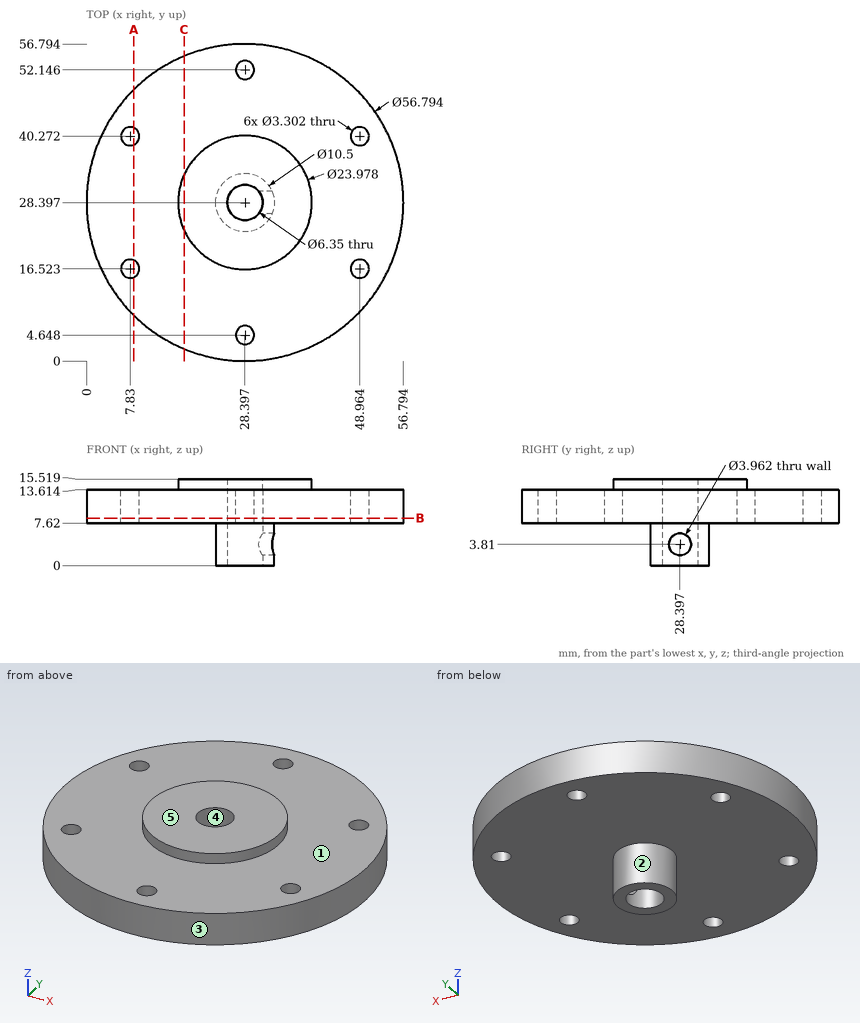
Part print with two shaded views. Sizes in mm from the minimum x, y, z corner. A direction names the side the tool comes from. Give positions to 0.01 mm unless a question says otherwise; leave off trailing zeros. Write each loop counter-clockwise with the first axis right and the second up, starting at its lowest first coordinate (ties: lowest second). Pieces come first, ordered by that corner, then holes.
1) Probe L1, parallel to Z at x = 20, y = 26; L2, parallel to Z at x = 35.5, y = 5 (1 decimal); L3, parallel to X at y = 27.5, z = 6.75 (1 decimal). List the from-to ranges inside material, lowest first.
Resolved:
L1: z = 7.62 to 15.52
L2: z = 7.6 to 13.6
L3: x = 23.2 to 25.4, 31.4 to 33.6
2) Two-plate mould, pull along Y, no slides. Class the marked faces 3, 4 and 5: released by +Y, released by -Y, zero draft, split by the parting line, or undercut.
Resolved:
face 3: split by the parting line
face 4: undercut
face 5: zero draft
3) Which spindle directions (+Z, -Z, +X, -X, +Y, -Y) get a long thin tool onto all of the face, cutting with end or side? Do the marked faces 1 and 2. Say none if no direction does.
Resolved:
face 1: +Z
face 2: -Z
4) Pin check, flat tips, straight feed: pin 1 (12 mm diameter, centred on x = 17, y = 15, fed in from -Z); pin 2 (1 mm diameter, centred on x = 46, z = 7.5, fed in from -Y); pin 3 (1.5 mm diameter, centred on x = 15, z = 8, fed in from -Y). Stop position of each tip, or through.
Resolved:
pin 1: stops at z = 7.62
pin 2: stops at y = 5.74
pin 3: stops at y = 2.97
5) Cut at B-B on z = 8.5. State how many separate pieces and enclosed holes the cut face has, then the cut area to 3 significant figures.
Resolved:
separate pieces: 1
enclosed holes: 7
area: 2,450 mm2
6) Cut at C-C on x = 17.5. Write the cut outline in (y, z) (1 decimal).
Resolved:
outline: (2.2, 7.6) - (54.6, 7.6) - (54.6, 13.6) - (33.4, 13.6) - (33.4, 15.5) - (23.4, 15.5) - (23.4, 13.6) - (2.2, 13.6) - close
7) Cut at A-A on x = 8.5. Write the cut outline in (y, z) (1 decimal), then the cut area to 3 significant figures.
Resolved:
outline: (8.1, 7.6) - (15, 7.6) - (15, 13.6) - (8.1, 13.6) - close; (18, 7.6) - (38.8, 7.6) - (38.8, 13.6) - (18, 13.6) - close; (41.8, 7.6) - (48.7, 7.6) - (48.7, 13.6) - (41.8, 13.6) - close
area: 207 mm2
